Input: part model. Units: mm. Frame: model coordinates. Face numbers are marked on the shaded views. A direction names the side the tool comes from. Give positions to 0.01 mm unless a question says otherwise; leave off trailing zeros. Loops run counter-clockwise (first coordinate to the right, second up) from the corner with the lowest first, then second, coordinate; pieces in that order, holes last.
from build123d import *

# Parameters (mm, degrees)
SKETCH1_W           = 65
SKETCH1_H           = 65
BOSS_EXTRUDE1_DEPTH = 30
SKETCH3_R           = 17.5
BOSS_EXTRUDE2_DEPTH = 15
SKETCH4_R           = 25
BOSS_EXTRUDE3_DEPTH = 70
SKETCH5_R           = 7.5
BOSS_EXTRUDE4_DEPTH = 3
SKETCH6_R           = 4
BOSS_EXTRUDE5_DEPTH = 10
SKETCH7_R           = 10
BOSS_EXTRUDE6_DEPTH = 30
CUT_EXTRUDE1_DEPTH  = 22.38


with BuildPart() as part:
    # Sketch1 → Boss-Extrude1 (new body)
    with BuildSketch(Plane(origin=(0, 0, 0), x_dir=(1, 0, 0), z_dir=(0, 1, 0))):
        Rectangle(SKETCH1_W, SKETCH1_H)
    extrude(amount=BOSS_EXTRUDE1_DEPTH)

    # Sketch3 → Boss-Extrude2 (add)
    with BuildSketch(Plane(origin=(0, 30, 0), x_dir=(1, 0, 0), z_dir=(0, 1, 0))):
        Circle(SKETCH3_R)
    extrude(amount=BOSS_EXTRUDE2_DEPTH)

    # Sketch4 → Boss-Extrude3 (add)
    with BuildSketch(Plane(origin=(0, 45, 0), x_dir=(1, 0, 0), z_dir=(0, 1, 0))):
        Circle(SKETCH4_R)
    extrude(amount=BOSS_EXTRUDE3_DEPTH)

    # Sketch5 → Boss-Extrude4 (add)
    with BuildSketch(Plane.XZ):
        with Locations((-12.500000122, 0.50000004)):
            Circle(SKETCH5_R)
    extrude(amount=BOSS_EXTRUDE4_DEPTH)

    # Sketch6 → Boss-Extrude5 (add)
    with BuildSketch(Plane.XZ.offset(3)):
        with Locations((-12.500000122, 0.50000004)):
            Circle(SKETCH6_R)
    extrude(amount=BOSS_EXTRUDE5_DEPTH)

    # Sketch7 → Boss-Extrude6 (add)
    with BuildSketch(Plane.XZ.offset(13)):
        with Locations((-12.500000122, 0.50000004)):
            Circle(SKETCH7_R)
    extrude(amount=BOSS_EXTRUDE6_DEPTH)

    # Sketch8 → Cut-Extrude1 (cut)
    with BuildSketch(Plane.XZ.offset(43)):
        with BuildLine():
            Line((-17.733861002, 3.106945343), (-7.140648736, 3.106945343))
            ThreePointArc((-7.140648736, 3.106945343), (-12.437254869, -3.029833946), (-17.733861002, 3.106945343))
        make_face()
    extrude(amount=-CUT_EXTRUDE1_DEPTH, mode=Mode.SUBTRACT)


solid = part.part
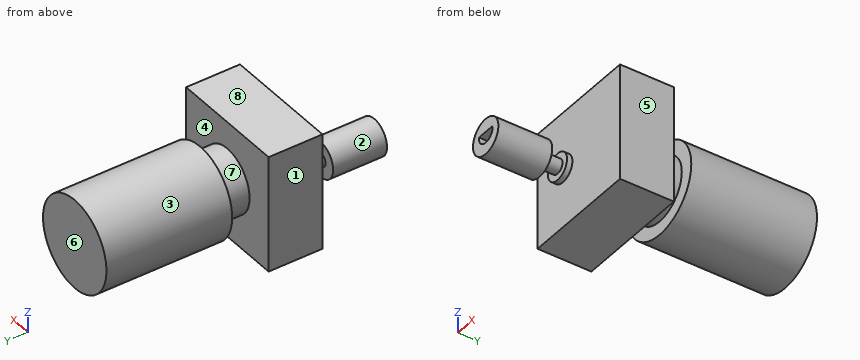
(1) Cut plane C-C (y = 41.5). Return the cut outline in (x, z).
Values follow:
outline: circle Ø35 at (0, 0)
(2) Pin query (flat end, axial travel): pin 1 Ø12 at (x, y) = (11, 79) entering from +Z; pin 2 Ø10 at (x, z) = (0, 15) entering from -Y; pin 3 Ø12 at (y, z) = (-15, -2.5) entering from -X. Return the tip coordinate at first contact, or that it passes through.
Values follow:
pin 1: stops at z = 24.49
pin 2: stops at y = 0
pin 3: stops at x = -22.5
(3) Mould query, pull axis Y, two halves, no side actions, for the marked faces 6, 7 and 8. Classes: +Y half, -Y half, draft (parallel to the pull), parting line (faces both ways), or undercut.
Values follow:
face 6: +Y half
face 7: undercut
face 8: draft
(4) Cut plane D-D (z = -23). Return the cut outline in (x, y), and give its area (3 significant figures).
Values follow:
outline: (-32.5, 0) - (32.5, 0) - (32.5, 30) - (-32.5, 30) - close; (-9.8, 45) - (9.8, 45) - (9.8, 115) - (-9.8, 115) - close
area: 3,320 mm2
(5) Cut plane A-A (z = 20). Return the cut outline in (x, y).
Values follow:
outline: (-32.5, 0) - (32.5, 0) - (32.5, 30) - (-32.5, 30) - close; (-15, 45) - (15, 45) - (15, 115) - (-15, 115) - close
(6) Ray query, probe 1 along Y at (x, z) = (-8.5, 9.5); probe 2 along Y at (x, z) = (10, -16); probe 3 along Y at (x, z) = (-4.5, 25). Return the intervals inside material, ascending.
Values follow:
probe 1: y = -43 to -13, 0 to 115
probe 2: y = 0 to 30, 45 to 115
probe 3: y = 0 to 30
(7) Cut plane B-B (x = -10). Return the cut outline in (y, z).
Values follow:
outline: (-43, -9.18) - (-13, -9.18) - (-13, -2.62) - (-3, -2.62) - (-3, -6.57) - (0, -6.57) - (0, -32.5) - (30, -32.5) - (30, -14.36) - (45, -14.36) - (45, -22.91) - (115, -22.91) - (115, 22.91) - (45, 22.91) - (45, 14.36) - (30, 14.36) - (30, 32.5) - (0, 32.5) - (0, 7.57) - (-3, 7.57) - (-3, 3.62) - (-13, 3.62) - (-13, 10.18) - (-43, 10.18) - (-43, 3.11) - (-20.62, 3.11) - (-20.62, -2.44) - (-43, -2.44) - close
(8) Reachability of the marked faces 1, 2, 3, 4 and 5 from +Z, -Z, +X, -X, +Y, -Y: full face, straight path, thin tool, end or side. Return the list, or none.
Values follow:
face 1: +Z, -Z, -X, +Y, -Y
face 2: -Y
face 3: +Y
face 4: none
face 5: +Z, -Z, +X, +Y, -Y
